Can you work these out from the model? Positions are in its coordinate system, mm. Face numbers are marked on the shaded views. A direction names the side the tool comes from. Coordinates: 2 decimals unless noted, no trailing zeros. Order: outer loops, then holes, each group sorted by start corner. A loop starts at its lowest first (then second) coordinate and runs counter-clockwise, first axis right, second up. Notation, with made-up numbers: (10, 68) - (51, 68) arc R25 ccw to (51, 80) - close; hole circle Ø3 at (15.5, 62). An arc over 180 degrees is marked (long way). Use a Markdown table: item, result. Add a question column.
(1) For pin 1 Ø3 at (y, z) = (6, -115) entering from -X; pin 2 Ø6 at (x, z) = (6, -112) entering from -Y; pin 3 Ø1.5 at (y, z) = (18, -117.5) entering from +X; pin 4 Ø4 at (x, y) = (13.5, 6.5) entering from -Z, each with a flat end and sliding along its axis, tell me the tip position at first contact or that it passes through.
(2) I want a section at A-A (x = 10). List the corners of the cut face in (y, z) for me, and give its area (3 significant figures).
(3) We'd pull the mould along Y, two halves only. Please class the marked faces 3, 4 and 5: pulls with the +Y half, pulls with the -Y half, needs draft (parallel to the pull), parting line crosses it, or undercut.
(4) On a 3-axis mill with a long thin cutter (end or side, diameter ignored), from which of +Z, -Z, +X, -X, +Y, -Y can I reach the whole of each face in a straight line? I mean the marked faces 1 and 2. Say none if no direction works.
(5) If I drill on L1, parallel to Z at x = 2, y = 8.75; L2, parallel to Z at x = 9.25, y = 6.5; L3, parallel to Y at x = 14, z = -122, over which ranges is the centre line in solid material (lowest first)? Write a range as [from, to].
(6) I want a section at D-D (z = -108.25). List the corners of the cut face in (x, y) for me, and give its area (3 significant figures).
(7) I want a section at C-C (z = -118.25). List the corners of the cut face in (x, y) for me.
```python
from build123d import *

# Parameters (mm, degrees)
CYLINDER003_R           = 10
CYLINDER003_DEPTH       = 15
CYLINDER004_R           = 5.5
CYLINDER004_DEPTH       = 10
CYLINDER005_R           = 5.5
CYLINDER005_DEPTH       = 11
BODY006_PLACEMENT_ANGLE = 90


with BuildPart() as part:
    # Cylinder003 → Cylinder003 (join)
    with BuildSketch(Plane(origin=(10, 0, -127), x_dir=(0, 1, 0), z_dir=(0, 0, 1))):
        Circle(CYLINDER003_R)
    extrude(amount=CYLINDER003_DEPTH)

    # Cylinder004 → Cylinder004 (join)
    with BuildSketch(Plane(origin=(10, 0, -112), x_dir=(1, 0, 0), z_dir=(0, 0, 1))):
        Circle(CYLINDER004_R)
    extrude(amount=CYLINDER004_DEPTH)

    # Cylinder005 → Cylinder005 (cut)
    with BuildSketch(Plane(origin=(10, 0, -127), x_dir=(1, 0, 0), z_dir=(0, 0, 1))):
        Circle(CYLINDER005_R)
    extrude(amount=CYLINDER005_DEPTH, mode=Mode.SUBTRACT)


with BuildPart() as part_1:
    # Body006 placement: moved
    add(part.part.moved(Location((10, 0, -1))).rotate(Axis((10, 0, -1), (0, 0, 1)), BODY006_PLACEMENT_ANGLE))


solid = part_1.part
```
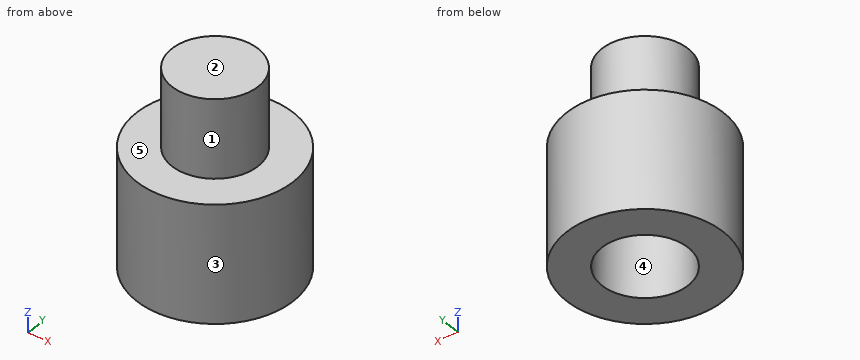
Answers follow:
| question | item | result |
|---|---|---|
| 1 | pin 1 | stops at x = 0.32 |
| 1 | pin 2 | stops at y = 0.07 |
| 1 | pin 3 | stops at x = 16.89 |
| 1 | pin 4 | stops at z = -128 |
| 2 | outline | (0, -128) - (4.5, -128) - (4.5, -117) - (15.5, -117) - (15.5, -128) - (20, -128) - (20, -113) - (15.5, -113) - (15.5, -103) - (4.5, -103) - (4.5, -113) - (0, -113) - close |
| 2 | area | 289 mm² |
| 3 | face 3 | parting line crosses it |
| 3 | face 4 | undercut |
| 3 | face 5 | needs draft |
| 4 | face 1 | +Z |
| 4 | face 2 | +Z, +X, -X, +Y, -Y |
| 5 | L1 | z = [-128, -113] |
| 5 | L2 | z = [-117, -103] |
| 5 | L3 | y = [0.83, 6.23], [13.77, 19.17] |
| 6 | outline | circle Ø11 at (10, 10) |
| 6 | area | 95.0 mm² |
| 7 | outline | circle Ø20 at (10, 10); hole circle Ø11 at (10, 10) |
